```python
from build123d import *

# Parameters (mm, degrees)
F0_R          = 20
F1_DEPTH      = 324
F1_DEPTH_BACK = 191
F3_DEPTH      = 5
F4_SIZE2      = 28.356399
F4_SIZE       = 4.99999


# Not quite as in the source:
# - a fillet or chamfer is up to 0.001 mm smaller than in the source, because OpenCascade refuses the exact size


with BuildPart() as f1:
    # F0 (on Top) → F1 (new body, two sides)
    with BuildSketch(Plane.XY) as f1_sk:
        Circle(F0_R)
    extrude(amount=F1_DEPTH)
    extrude(f1_sk.sketch, amount=-F1_DEPTH_BACK)

    # F2 (on Right) → F3 (join)
    with BuildSketch(Plane.YZ):
        with BuildLine():
            Line((9.8391985521, 165.7918989658), (21.8501202762, 166.5147198653))
            Line((21.8501202762, 166.5147198653), (172.5762003339, 47.3351646042))
            ThreePointArc((172.5762003339, 47.3351646042), (231.5665738369, 202.382288244), (172.5762003339, 357.4294118838))
            Line((172.5762003339, 357.4294118838), (22.4253297422, 237.5259771443))
            Line((22.4253297422, 237.5259771443), (9.8391985521, 237.5259771443))
            Line((9.8391985521, 237.5259771443), (9.8391985521, 165.7918989658))
        make_face()
    extrude(amount=F3_DEPTH)

    # F4 (size 5 and 28.3564090981 in the source; OpenCascade refuses exactly that, so slightly less here)
    f4_edges = [f1.edges().sort_by_distance(p)[0] for p in [
        (5, 231.566574, 202.382288),
    ]]
    f4_side = f1.faces().sort_by_distance((2.5, 231.566574, 202.382288))[0]
    chamfer(f4_edges, length=F4_SIZE, length2=F4_SIZE2, reference=f4_side)

    # F5: F1 across plane


with BuildPart() as f1_1:
    add(f1.part)
    add(f1.part.mirror(Plane.YZ))

    # F6: F1 across plane


with BuildPart() as f1_2:
    add(f1_1.part)
    add(f1_1.part.mirror(Plane.XZ))

    # F7 (on Right) → F8 (revolve)
    with BuildSketch(Plane.YZ):
        Polygon((5.505359266, 312.6185536385), (5.505359266, 329.4300734997), (19.3500220776, 329.4300734997), (0, 373.1769025326), (0, 329.4300734997), (0, 312.6185536385), align=None)
    revolve(axis=Axis((0, 0, 351.3034880161), (0, 0, -1)))

    # F9 (on Right) → F10 (revolve)
    with BuildSketch(Plane.YZ):
        with BuildLine():
            Line((-15.0489732623, -187.7072155476), (-15.0489732623, -192.4124807119))
            Line((-15.0489732623, -192.4124807119), (-23.5689829473, -209.4524800777))
            ThreePointArc((-23.5689829473, -209.4524800777), (-12.5456612149, -215.444084642), (0, -215.3050452471))
            Line((0, -215.3050452471), (0, -209.4524800777))
            Line((0, -209.4524800777), (0, -193.2779252529))
            Line((0, -193.2779252529), (0, -187.7072155476))
            Line((0, -187.7072155476), (-15.0489732623, -187.7072155476))
        make_face()
    revolve(axis=Axis((0, 0, -201.3652026653), (0, 0, -1)))


solid = f1_2.part
```
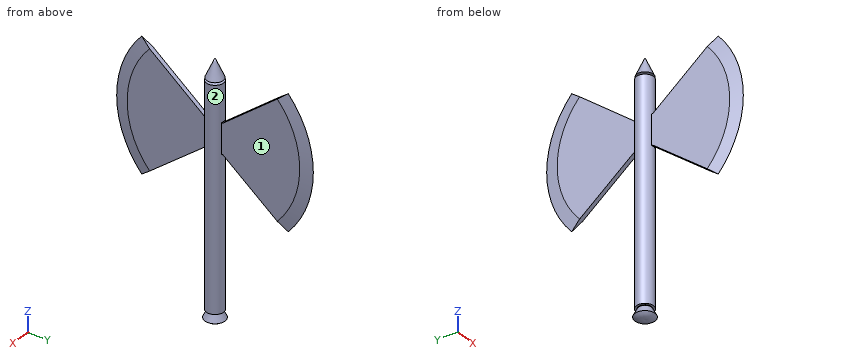
Verification items for the finished model (mm, model axes). Face numbers are marked on the shaded views. Give positions to 0.01 mm unless a question says otherwise; leave off trailing zeros. Order: outer loops, then holes, each group sorted by start corner. A loop starts at its lowest first (then second) coordinate and runs counter-clockwise, first axis right, second up. Notation, with made-up numbers: M 20,83 L 60,83 A19 cw 60,93 Z; hole C 45,68.25 d4. An arc over 180 degrees is marked long. Answer in a Markdown table with one row per item. Add a question column.
Item 1: Mould release check, pull along Z, two halves, no side actions. Record for the marked faces 1 and 2: released by +Z, released by -Z, zero draft, split by the parting line, or undercut.
Item 2: Section check A-A, the plane z = -70.5. Enter the section's corners in (x, y), and give its area (3 significant figures).
Item 3: Section check D-D, the plane y = -34. Enter the section's corners in (x, z).
Item 4: Section check C-C, the plane z = 88.5. State how many separate pieces and enclosed holes the cut face has, and give its area (3 significant figures).
Item 5: Section check B-B, the plane y = 82. Enter the section's corners in (x, z), and give its area (3 significant figures).
Item 6: Scan lines: probe 1 along X at (y, z) = (-130.5, 137.5); probe 2 along Y at (x, z) = (12.5, -107); probe 3 along Y at (x, z) = (11, 241.5). Record each from-to range of solid material in increasing order. Write a range as from..to.
Item 7: Gauge pin test, flat ends, axial feed: pin 1 (2 mm diameter, centred on y = 25, z = 222, fed in from +X); pin 2 (1.5 mm diameter, centred on x = -1.5, y = 20.5, fed in from +Z); pin 3 (10 mm diameter, centred on x = -2.5, z = -74.5, fed in from -Y). Record the tip position at first contact, or that the pin passes through.
Filled sheet:
| question | item | result |
|---|---|---|
| 1 | face 1 | zero draft |
| 1 | face 2 | undercut |
| 2 | outline | C 0,0 d40 |
| 2 | area | 1,260 mm^2 |
| 3 | outline | M -5,156.91 L 5,156.91 L 5,246.77 L -5,246.77 Z |
| 4 | separate pieces | 3 |
| 4 | enclosed holes | 0 |
| 4 | area | 2,550 mm^2 |
| 5 | outline | M -5,118.95 L 5,118.95 L 5,285.1 L -5,285.1 Z |
| 5 | area | 1,660 mm^2 |
| 6 | probe 1 | x = -5..5 |
| 6 | probe 2 | y = -15.61..15.61 |
| 6 | probe 3 | y = -16.7..16.7 |
| 7 | pin 1 | stops at x = 5 |
| 7 | pin 2 | stops at z = 324 |
| 7 | pin 3 | stops at y = -20 |
